from build123d import *

# Parameters (mm, degrees)
BOSS_EXTRU_1_DEPTH      = 14
ESQUISSE2_W             = 7.5
ESQUISSE2_H             = 6
ESQUISSE2_W_2           = 15
ESQUISSE2_W_3           = 10
ESQUISSE2_H_2           = 4
ENL_V_MAT_EXTRU_1_DEPTH = 15


with BuildPart() as part:
    # Esquisse1 → Boss.-Extru.1 (new body)
    with BuildSketch(Plane.XY):
        with BuildLine():
            ThreePointArc((7.5, 7.5), (5.303300859, 2.196699141), (0, 0))
            Line((0, 0), (45, 0))
            ThreePointArc((45, 0), (37.5, 7.5), (45, 15))
            Line((45, 15), (0, 15))
            ThreePointArc((0, 15), (5.303300859, 12.803300859), (7.5, 7.5))
        make_face()
        with BuildLine():
            ThreePointArc((45, 15), (37.5, 7.5), (45, 0))
            Line((45, 0), (45, 2.5))
            ThreePointArc((45, 2.5), (40, 7.5), (45, 12.5))
            Line((45, 12.5), (45, 15))
        make_face()
        with BuildLine():
            Line((45, 2.5), (45, 0))
            ThreePointArc((45, 0), (50.303300859, 2.196699141), (52.5, 7.5))
            ThreePointArc((52.5, 7.5), (50.303300859, 12.803300859), (45, 15))
            Line((45, 15), (45, 12.5))
            ThreePointArc((45, 12.5), (48.535533906, 11.035533906), (50, 7.5))
            ThreePointArc((50, 7.5), (48.535533906, 3.964466094), (45, 2.5))
        make_face()
        with BuildLine():
            ThreePointArc((0, 15), (-7.5, 7.5), (0, 0))
            Line((0, 0), (0, 2.5))
            ThreePointArc((0, 2.5), (-5, 7.5), (0, 12.5))
            Line((0, 12.5), (0, 15))
        make_face()
        with BuildLine():
            Line((0, 2.5), (0, 0))
            ThreePointArc((0, 0), (5.303300859, 2.196699141), (7.5, 7.5))
            ThreePointArc((7.5, 7.5), (5.303300859, 12.803300859), (0, 15))
            Line((0, 15), (0, 12.5))
            ThreePointArc((0, 12.5), (3.535533906, 11.035533906), (5, 7.5))
            ThreePointArc((5, 7.5), (3.535533906, 3.964466094), (0, 2.5))
        make_face()
    extrude(amount=BOSS_EXTRU_1_DEPTH)

    # Esquisse2 → Enlèv. mat.-Extru.1 (cut)
    with BuildSketch(Plane(origin=(0, 15, 0), x_dir=(1, 0, 0), z_dir=(0, 1, 0))):
        with Locations((-3.75, -7)):
            Rectangle(ESQUISSE2_W, ESQUISSE2_H)
        with Locations((7.5, -7)):
            Rectangle(ESQUISSE2_W_2, ESQUISSE2_H)
        with Locations((40, -2)):
            Rectangle(ESQUISSE2_W_3, ESQUISSE2_H_2)
        with Locations((48.75, -2)):
            Rectangle(ESQUISSE2_W, ESQUISSE2_H_2)
        with Locations((48.75, -12)):
            Rectangle(ESQUISSE2_W, ESQUISSE2_H_2)
        with Locations((40, -12)):
            Rectangle(ESQUISSE2_W_3, ESQUISSE2_H_2)
    extrude(amount=-ENL_V_MAT_EXTRU_1_DEPTH, mode=Mode.SUBTRACT)


solid = part.part
Work out the finished part from the listing and answer in its coordinate system (mm). A direction names the side the tool comes from. Give positions to 0.01 mm unless a question says otherwise; leave off trailing zeros. Order: outer loops, then holes, each group sorted by start corner. A loop starts at its lowest first (then second) coordinate and runs counter-clockwise, first axis right, second up. Notation, with made-up numbers: M 14.5,12 L 55.5,12 A17 cw 55.5,42 Z; hole C 24,80 d10. An arc over 180 degrees is marked long. Return JSON: item names as keys, results as strings.
Q1. Each of these flat-tipped pins is pushed along its axis until it touches: pin 1 (3 mm diameter, centred on y = 5.5, z = 12.5, fed in from +X); pin 2 (4.5 mm diameter, centred on y = 7, z = 2, fed in from +X); pin 3 (1 mm diameter, centred on x = 41, y = 11.5, fed in from -Z); pin 4 (4 mm diameter, centred on y = 11, z = 4, fed in from +X). Where does it stop, or does it pass through?
Answer below:
{"pin 1": "stops at x = 35", "pin 2": "stops at x = 52.5", "pin 3": "stops at z = 4", "pin 4": "stops at x = 52.35"}
Q2. Which of the six approach directions +Z, -Z, +X, -X, +Y, -Y give full straight-line access (tool end or side, diameter ignored) to faces 4 (the face through (6, 8, 10)), 5 (the face through (35, 8, 2)), 6 (the face through (40, 9, 10))?
Answer below:
{"face 4": "-X, +Y, -Y", "face 5": "-Z, +X, +Y, -Y", "face 6": "+Z, +X, +Y, -Y"}
Q3. Find section D-D, the plane y = 1.25. Write down the section's boundary in (x, z), and give its area (3 significant figures).
Answer below:
{"outline": "M -4.15,0 L 35,0 L 35,4 L 49.15,4 L 49.15,10 L 35,10 L 35,14 L -4.15,14 L -4.15,10 L 15,10 L 15,4 L -4.15,4 Z", "area": "518 mm^2"}
Q4. Find section A-A, the plane z = 2.75. Write down the section's boundary in (x, y).
Answer below:
{"outline": "M 0,0 L 35,0 L 35,15 L 0,15 A7.5 ccw Z; hole C 0,7.5 d10"}
Q5. Find section B-B, the plane y = 5.75. Write down the section's boundary in (x, z), and give its area (3 significant figures).
Answer below:
{"outline": "M -7.29,0 L -4.68,0 L -4.68,4 L -7.29,4 Z; M -7.29,10 L -4.68,10 L -4.68,14 L -7.29,14 Z; M 4.68,0 L 35,0 L 35,4 L 40.32,4 L 40.32,10 L 35,10 L 35,14 L 4.68,14 L 4.68,10 L 15,10 L 15,4 L 4.68,4 Z; M 49.68,4 L 52.29,4 L 52.29,10 L 49.68,10 Z", "area": "431 mm^2"}
Q6. The mould has two halves that part along Z. Classify faces 1 (the face through (15, 8, 7)), 2 (the face through (39.7, 7.6, 4)), 3 (the face through (22, 0, 7)): pulls with the +Z half, pulls with the -Z half, needs draft (parallel to the pull), parting line crosses it, or undercut.
Answer below:
{"face 1": "undercut", "face 2": "pulls with the -Z half", "face 3": "needs draft"}
Q7. Find the intervals of material crossed by line 1 along X through (y, z) = (7.5, 6); line 2 along Z through (x, y) = (12.5, 11); line 3 along X through (y, z) = (7.25, 11.25), in increasing order. Write a range as [from, to].
Answer below:
{"line 1": "x = [15, 40], [50, 52.5]", "line 2": "z = [0, 4], [10, 14]", "line 3": "x = [-7.5, -4.99], [4.99, 35]"}
Q8. Find section C-C, the plane x = 47. Write down the section's boundary in (y, z).
Answer below:
{"outline": "M 0.27,4 L 2.92,4 L 2.92,10 L 0.27,10 Z; M 12.08,4 L 14.73,4 L 14.73,10 L 12.08,10 Z"}
